For this review, take the finished solid that the model builds, in its own axes (mm). Round coordinates to 2 decimals unless told otherwise and drop trailing zeros. Write each loop counter-clockwise with the first axis right and the second up, starting at its lowest first coordinate (ties: lowest second). Pieces come first, ordered by that corner, then holes. Notation, with made-up numbers: (37.25, 47.25) -> (42.25, 47.25) arc R18 cw to (42.25, 53.25) -> close; hole circle Ø2 at (-12, -37). An arc over 180 degrees is marked (long way). Answer in a Markdown table with one row per item. Add a question column.
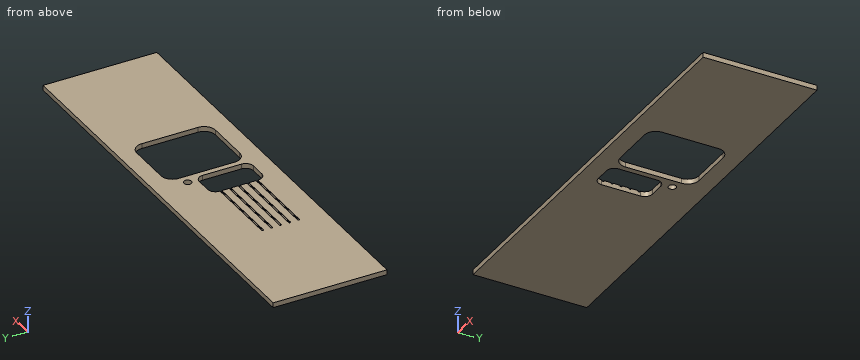
```python
from build123d import *

# Parameters (mm, degrees)
F0_W     = 2190
F0_H     = 600
F1_DEPTH = 26
F3_DEPTH = 26.001
F5_DEPTH = 6
F6_R     = 3
F7_R     = 20
F8_DEPTH = 26.001


with BuildPart() as f1:
    # F0 (on Top) → F1 (new body)
    with BuildSketch(Plane.XY):
        Rectangle(F0_W, F0_H)
    extrude(amount=F1_DEPTH)

    # F2 (on face) → F3 (cut, through all)
    with BuildSketch(Plane.XY.offset(26)):
        with BuildLine():
            Line((135, -205), (365, -205))
            ThreePointArc((365, -205), (407.426407, -187.426407), (425, -145))
            Line((425, -145), (425, 150))
            ThreePointArc((425, 150), (407.426407, 192.426407), (365, 210))
            Line((365, 210), (135, 210))
            ThreePointArc((135, 210), (92.573593, 192.426407), (75, 150))
            Line((75, 150), (75, -145))
            ThreePointArc((75, -145), (92.573593, -187.426407), (135, -205))
        make_face()
        with BuildLine():
            Line((-75, -205), (5, -205))
            ThreePointArc((5, -205), (33.284271, -193.284271), (45, -165))
            Line((45, -165), (45, 40))
            ThreePointArc((45, 40), (33.284271, 68.284271), (5, 80))
            Line((5, 80), (-75, 80))
            ThreePointArc((-75, 80), (-103.284271, 68.284271), (-115, 40))
            Line((-115, 40), (-115, -165))
            ThreePointArc((-115, -165), (-103.284271, -193.284271), (-75, -205))
        make_face()
    extrude(amount=-F3_DEPTH, mode=Mode.SUBTRACT)

    # F4 (on face) → F5 (cut)
    with BuildSketch(Plane.XY.offset(26)):
        with BuildLine():
            Line((-115, -162.5), (-115, -152.5))
            Line((-115, -152.5), (-512, -152.5))
            ThreePointArc((-512, -152.5), (-514.12132, -153.37868), (-515, -155.5))
            Line((-515, -155.5), (-515, -159.5))
            ThreePointArc((-515, -159.5), (-514.12132, -161.62132), (-512, -162.5))
            Line((-512, -162.5), (-115, -162.5))
        make_face()
        with BuildLine():
            Line((-115, -115), (-115, -105))
            Line((-115, -105), (-512, -105))
            ThreePointArc((-512, -105), (-514.12132, -105.87868), (-515, -108))
            Line((-515, -108), (-515, -112))
            ThreePointArc((-515, -112), (-514.12132, -114.12132), (-512, -115))
            Line((-512, -115), (-115, -115))
        make_face()
        with BuildLine():
            Line((-115, -67.5), (-115, -57.5))
            Line((-115, -57.5), (-512, -57.5))
            ThreePointArc((-512, -57.5), (-514.12132, -58.37868), (-515, -60.5))
            Line((-515, -60.5), (-515, -64.5))
            ThreePointArc((-515, -64.5), (-514.12132, -66.62132), (-512, -67.5))
            Line((-512, -67.5), (-115, -67.5))
        make_face()
        with BuildLine():
            Line((-115, -20), (-115, -10))
            Line((-115, -10), (-512, -10))
            ThreePointArc((-512, -10), (-514.12132, -10.87868), (-515, -13))
            Line((-515, -13), (-515, -17))
            ThreePointArc((-515, -17), (-514.12132, -19.12132), (-512, -20))
            Line((-512, -20), (-115, -20))
        make_face()
        with BuildLine():
            Line((-115, 27.5), (-115, 37.5))
            Line((-115, 37.5), (-512, 37.5))
            ThreePointArc((-512, 37.5), (-514.12132, 36.62132), (-515, 34.5))
            Line((-515, 34.5), (-515, 30.5))
            ThreePointArc((-515, 30.5), (-514.12132, 28.37868), (-512, 27.5))
            Line((-512, 27.5), (-115, 27.5))
        make_face()
    extrude(amount=-F5_DEPTH, mode=Mode.SUBTRACT)

    # F6
    f6_edges = [f1.edges().sort_by_distance(p)[0] for p in [
        (-313.5, 37.5, 20),
        (-313.5, -10, 20),
        (-313.5, -57.5, 20),
        (-313.5, -105, 20),
        (-313.5, -152.5, 20),
        (-313.5, -162.5, 20),
        (-313.5, -115, 20),
        (-313.5, -20, 20),
        (-313.5, -67.5, 20),
        (-313.5, 27.5, 20),
    ]]
    fillet(f6_edges, radius=F6_R)

    # F7 (on face) → F8 (cut, through all)
    with BuildSketch(Plane.XY.offset(26)):
        with Locations((25, 130)):
            Circle(F7_R)
    extrude(amount=-F8_DEPTH, mode=Mode.SUBTRACT)


solid = f1.part
```
1. We need section A-A (y = 130). Write out the cut boundary in (x, z), plus the area to 3 significant figures.
2. We need section C-C (x = 161.5). Write out the cut boundary in (y, z).
3. Clearance check with a flat-ended pin moving along its axis: pin 1 Ø1.2 at (x, y) = (-376, -62) entering from +Z. State where the tip first meets the part, or that it passes through.
4. We need section B-B (z = 8). Write out the cut boundary in (x, y), plus the area to 3 significant figures.
5. For L1, parallel to X at y = -71.5, z = 2.5; L2, parallel to Y at x = -389, z = 23; L3, parallel to X at y = 144.5, z = 23, list the stretches that pass through material, from the lowest coordinate up. Write a range as [from, to].
Response:
| question | item | result |
|---|---|---|
| 1 | outline | (-1095, 0) -> (5, 0) -> (5, 26) -> (-1095, 26) -> close; (45, 0) -> (75, 0) -> (75, 26) -> (45, 26) -> close; (425, 0) -> (1095, 0) -> (1095, 26) -> (425, 26) -> close |
| 1 | area | 46,800 mm2 |
| 2 | outline | (-300, 0) -> (-205, 0) -> (-205, 26) -> (-300, 26) -> close; (210, 0) -> (300, 0) -> (300, 26) -> (210, 26) -> close |
| 3 | pin 1 | z = 20 |
| 4 | outline | (-1095, -300) -> (1095, -300) -> (1095, 300) -> (-1095, 300) -> close; hole (-115, -165) arc R40 ccw to (-75, -205) -> (5, -205) arc R40 ccw to (45, -165) -> (45, 40) arc R40 ccw to (5, 80) -> (-75, 80) arc R40 ccw to (-115, 40) -> close; hole circle Ø40 at (25, 130); hole (75, -145) arc R60 ccw to (135, -205) -> (365, -205) arc R60 ccw to (425, -145) -> (425, 150) arc R60 ccw to (365, 210) -> (135, 210) arc R60 ccw to (75, 150) -> close |
| 4 | area | 1,130,000 mm2 |
| 5 | L1 | [-1095, -115], [45, 75], [425, 1095] |
| 5 | L2 | [-300, -162.5], [-152.5, -115], [-105, -67.5], [-57.5, -20], [-10, 27.5], [37.5, 300] |
| 5 | L3 | [-1095, 11.23], [38.77, 75], [425, 1095] |
